For this review, take the finished solid that the model builds, in its own axes (mm). Face numbers are marked on the shaded views. A direction names the side the tool comes from. Give positions to 0.01 mm unless a question says otherwise; leave off trailing zeros. Write each loop counter-clockwise with the first axis right and the second up, starting at its lowest first coordinate (ties: lowest second). Pieces come first, ordered by that corner, then holes.
Q1. Insertion check: P1, Ø3.5, axis at x = 0, y = 0, coming from the +Z side; P2, Ø4, axis at x = 10, y = -9.5, coming from the +Z side; P3, Ø2, axis at y = -10, z = 6.5, coming from the +X side. Each pin has a flat end and moves straight along its axis. Give the tip position at first contact, or say it passes through.
Q2. Mouldability with a two-part tool opening along X and no side actions: class the marked faces 1, 2, 3 and 4 as released by +X, released by -X, zero draft, split by the parting line, or undercut.
Q3. We need section B-B (z = 14.25). Write out the cut boundary in (x, y), then the cut area to 3 significant figures.
Q4. Machinability: for the marked faces 5, 6, 7, 8 and 9, which of the approach directions +Z, -Z, +X, -X, +Y, -Y give a long, thin tool a straight path to every point of the face, cutting with its end or side? Answer none if there is none.
Q5. We need section D-D (z = 2). Write out the cut boundary in (x, y).
Q6. For line 1 (Z direction, x = 8, y = 4.25); line 2 (Z direction, x = 11.5, y = -5.5); line 3 (Y direction, x = -1, z = 2), list the stretches that pass through material, from the lowest coordinate up.
Q7. We need section A-A (x = 0). Write out the cut boundary in (y, z), then the cut area to 3 significant figures.
```python
from build123d import *

# Parameters (mm, degrees)
SCHIZZO1_W                            = 25
SCHIZZO1_H                            = 25
ESTRUSIONE_ESTRUSIONE1_DEPTH          = 8
SCHIZZO8_R                            = 5
ESTRUSIONE_ESTRUSIONE3_DEPTH          = 15
RACCORDO1_R                           = 3
TAGLIO_ESTRUSIONE2_REACH              = 25
SCHIZZO9_R                            = 1.6
SCHIZZO10_R                           = 3
TAGLIO_ESTRUSIONE3_DEPTH              = 4
SCHIZZO11_R                           = 3
TAGLIO_ESTRUSIONE4_DEPTH              = 16
TAGLIO_ESTRUSIONE6_REACH              = 25
SCHIZZO13_R                           = 1.6
TAGLIO_ESTRUSIONE8_START              = -3
TAGLIO_ESTRUSIONE8_DEPTH              = 19
RIPETIZIONECIRCOLARE1_COUNT           = 2
RIPETIZIONECIRCOLARE1_ANGLE           = 180
TAGLIO_ESTRUSIONE9_REACH              = 10
RACCORDO2_R                           = 5
RACCORDO3_R                           = 3
TAGLIO_ESTRUSIONE10_REACH             = 10
TAGLIO_ESTRUSIONE10_DIRECTION_2_REACH = 17


with BuildPart() as part:
    # Schizzo1 → Estrusione-Estrusione1 (new body)
    with BuildSketch(Plane.XY):
        Rectangle(SCHIZZO1_W, SCHIZZO1_H)
    extrude(amount=ESTRUSIONE_ESTRUSIONE1_DEPTH)

    # Schizzo8 → Estrusione-Estrusione3 (add)
    with BuildSketch(Plane.XY.offset(8)):
        Circle(SCHIZZO8_R)
    extrude(amount=ESTRUSIONE_ESTRUSIONE3_DEPTH)

    # Raccordo1
    raccordo1_edges = [part.edges().sort_by_distance(p)[0] for p in [
        (-5, 0, 8),
    ]]
    fillet(raccordo1_edges, radius=RACCORDO1_R)

    # Schizzo9 → Taglio-Estrusione2 (cut, up to next)
    with BuildSketch(Plane(origin=(0, 0, 0), x_dir=(-1, 0, 0), z_dir=(0, 0, -1)), mode=Mode.PRIVATE) as taglio_estrusione2_sk1:
        Circle(SCHIZZO9_R)
    taglio_estrusione2_tool1 = extrude(taglio_estrusione2_sk1.sketch, amount=-TAGLIO_ESTRUSIONE2_REACH, mode=Mode.PRIVATE) & part.part
    add(taglio_estrusione2_tool1.solids().sort_by_distance((0, 0, 0))[0], mode=Mode.SUBTRACT)

    # Schizzo10 → Taglio-Estrusione3 (cut)
    with BuildSketch(Plane(origin=(0, 0, 0), x_dir=(-1, 0, 0), z_dir=(0, 0, -1))):
        Circle(SCHIZZO10_R)
    extrude(amount=-TAGLIO_ESTRUSIONE3_DEPTH, mode=Mode.SUBTRACT)

    # Schizzo11 → Taglio-Estrusione4 (cut)
    with BuildSketch(Plane.XY.offset(23)):
        Circle(SCHIZZO11_R)
    extrude(amount=-TAGLIO_ESTRUSIONE4_DEPTH, mode=Mode.SUBTRACT)

    # Schizzo13 → Taglio-Estrusione6 (cut, up to next)
    with BuildSketch(Plane(origin=(0, 0, 0), x_dir=(-1, 0, 0), z_dir=(0, 0, -1)), mode=Mode.PRIVATE) as taglio_estrusione6_sk1:
        with Locations((-8.485281374, -8.485281374)):
            Circle(SCHIZZO13_R)
    taglio_estrusione6_tool1 = extrude(taglio_estrusione6_sk1.sketch, amount=-TAGLIO_ESTRUSIONE6_REACH, mode=Mode.PRIVATE) & part.part
    add(taglio_estrusione6_tool1.solids().sort_by_distance((8.485281, -8.485281, 0))[0], mode=Mode.SUBTRACT)
    # Schizzo13 → Taglio-Estrusione6 (cut, up to next)
    with BuildSketch(Plane(origin=(0, 0, 0), x_dir=(-1, 0, 0), z_dir=(0, 0, -1)), mode=Mode.PRIVATE) as taglio_estrusione6_sk2:
        with Locations((8.485281374, 8.485281374)):
            Circle(SCHIZZO13_R)
    taglio_estrusione6_tool2 = extrude(taglio_estrusione6_sk2.sketch, amount=-TAGLIO_ESTRUSIONE6_REACH, mode=Mode.PRIVATE) & part.part
    add(taglio_estrusione6_tool2.solids().sort_by_distance((-8.485281, 8.485281, 0))[0], mode=Mode.SUBTRACT)

    # Schizzo17 → Taglio-Estrusione8 (cut)
    with BuildSketch(Plane.XY.offset(8).offset(TAGLIO_ESTRUSIONE8_START)):
        with BuildLine():
            Line((4.5, -12.5), (4.5, -8.5))
            ThreePointArc((4.5, -8.5), (5.671572875, -5.671572875), (8.5, -4.5))
            Line((8.5, -4.5), (12.5, -4.5))
            Line((12.5, -4.5), (12.5, -12.5))
            Line((12.5, -12.5), (4.5, -12.5))
        make_face()
    taglio_estrusione8 = extrude(amount=TAGLIO_ESTRUSIONE8_DEPTH, mode=Mode.SUBTRACT)

    # RipetizioneCircolare1: Taglio-Estrusione8 ×2 about axis
    ripetizionecircolare1_axis = Axis((0, 0, 0), (0, 0, 1))
    for i in range(1, RIPETIZIONECIRCOLARE1_COUNT):
        add(taglio_estrusione8.rotate(ripetizionecircolare1_axis, i * RIPETIZIONECIRCOLARE1_ANGLE / (RIPETIZIONECIRCOLARE1_COUNT - 1)), mode=Mode.SUBTRACT)

    # Schizzo18 → Taglio-Estrusione9 (cut, up to next)
    with BuildSketch(Plane.XY.offset(8), mode=Mode.PRIVATE) as taglio_estrusione9_sk1:
        Polygon((2.5, 12.5), (12.5, 2.5), (12.5, 12.5), align=None)
    taglio_estrusione9_tool1 = extrude(taglio_estrusione9_sk1.sketch, amount=-TAGLIO_ESTRUSIONE9_REACH, mode=Mode.PRIVATE) & part.part
    add(taglio_estrusione9_tool1.solids().sort_by_distance((9.166667, 9.166667, 8))[0], mode=Mode.SUBTRACT)

    # Raccordo2
    raccordo2_edges = [part.edges().sort_by_distance(p)[0] for p in [
        (2.5, 12.5, 4),
        (12.5, 2.5, 4),
    ]]
    fillet(raccordo2_edges, radius=RACCORDO2_R)

    # Raccordo3
    raccordo3_edges = [part.edges().sort_by_distance(p)[0] for p in [
        (12.5, -12.5, 2.5),
        (-12.5, 12.5, 2.5),
    ]]
    fillet(raccordo3_edges, radius=RACCORDO3_R)

    # Schizzo19 → Taglio-Estrusione10 (cut, up to next)
    with BuildSketch(Plane.XY.offset(8), mode=Mode.PRIVATE) as taglio_estrusione10_sk1:
        with BuildLine():
            Line((4.5, -12.5), (6.885281374, -12.5))
            Line((6.885281374, -12.5), (-1.022619302, -7.934371416))
            ThreePointArc((-1.022619302, -7.934371416), (-4.933470073, -4.933470073), (-7.934371416, -1.022619302))
            Line((-7.934371416, -1.022619302), (-12.5, 6.885281374))
            Line((-12.5, 6.885281374), (-12.5, 4.5))
            Line((-12.5, 4.5), (-12.5, -12.5))
            Line((-12.5, -12.5), (4.5, -12.5))
        make_face()
    taglio_estrusione10_tool1 = extrude(taglio_estrusione10_sk1.sketch, amount=-TAGLIO_ESTRUSIONE10_REACH, mode=Mode.PRIVATE) & part.part
    add(taglio_estrusione10_tool1.solids().sort_by_distance((-6.87454, -6.87454, 8))[0], mode=Mode.SUBTRACT)

    # Schizzo19 → Taglio-Estrusione10 direction 2 (cut, up to next)
    with BuildSketch(Plane.XY.offset(8), mode=Mode.PRIVATE) as taglio_estrusione10_direction_2_sk1:
        with BuildLine():
            Line((4.5, -12.5), (6.885281374, -12.5))
            Line((6.885281374, -12.5), (-1.022619302, -7.934371416))
            ThreePointArc((-1.022619302, -7.934371416), (-4.933470073, -4.933470073), (-7.934371416, -1.022619302))
            Line((-7.934371416, -1.022619302), (-12.5, 6.885281374))
            Line((-12.5, 6.885281374), (-12.5, 4.5))
            Line((-12.5, 4.5), (-12.5, -12.5))
            Line((-12.5, -12.5), (4.5, -12.5))
        make_face()
    taglio_estrusione10_direction_2_tool1 = extrude(taglio_estrusione10_direction_2_sk1.sketch, amount=TAGLIO_ESTRUSIONE10_DIRECTION_2_REACH, mode=Mode.PRIVATE) & part.part
    add(taglio_estrusione10_direction_2_tool1.solids().sort_by_distance((-6.87454, -6.87454, 8))[0], mode=Mode.SUBTRACT)


solid = part.part
```
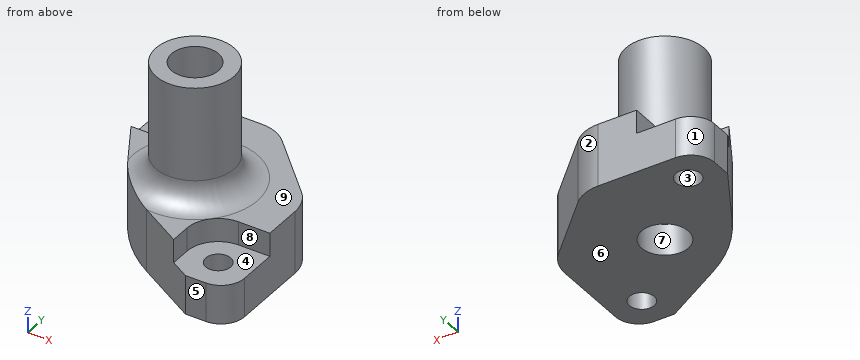
Computed:
1. P1: stops at z = 7
1. P2: stops at z = 5
1. P3: stops at x = 4.5
2. face 1: released by -X
2. face 2: released by +X
2. face 3: undercut
2. face 4: zero draft
3. outline: circle Ø10 at (0, 0); hole circle Ø6 at (0, 0)
3. area: 50.3 mm2
4. face 5: +Z, -Z, +X, -X, -Y
4. face 6: -Z, +X, -X, +Y, -Y
4. face 7: -Z
4. face 8: +Z, +X, -Y
4. face 9: +Z
5. outline: (-12.5, 6.89) - (-7.93, -1.02) arc R18.88 ccw to (-1.02, -7.93) - (6.89, -12.5) - (9.5, -12.5) arc R3 ccw to (12.5, -9.5) - (12.5, 0.43) arc R5 ccw to (11.04, 3.96) - (3.96, 11.04) arc R5 ccw to (0.43, 12.5) - (-9.5, 12.5) arc R3 ccw to (-12.5, 9.5) - close; hole circle Ø3.2 at (-8.49, 8.49); hole circle Ø6 at (0, 0); hole circle Ø3.2 at (8.49, -8.49)
6. line 1: z = 0 to 8
6. line 2: z = 0 to 5
6. line 3: y = -7.95 to -2.83, 2.83 to 12.5
7. outline: (-8.52, 0) - (-3, 0) - (-3, 4) - (-1.6, 4) - (-1.6, 7) - (-3, 7) - (-3, 23) - (-5, 23) - (-5, 11) arc R3 cw to (-8, 8) - (-8.52, 8) - close; (1.6, 4) - (3, 4) - (3, 0) - (12.5, 0) - (12.5, 8) - (8, 8) arc R3 cw to (5, 11) - (5, 23) - (3, 23) - (3, 7) - (1.6, 7) - close
7. area: 192 mm2
